```python
from build123d import *

# Parameters (mm, degrees)
BOSS_EXTRUDE1_DEPTH       = 95
SKETCH4_W                 = 5
SKETCH4_H                 = 5
BOSS_EXTRUDE4_DEPTH       = 2
FILLET1_R                 = 1.5875
F_0_80_TAPPED_HOLE1_D     = 1.19126
F_0_80_TAPPED_HOLE1_DEPTH = 4.0005
F_0_80_TAPPED_HOLE1_TIP   = 0.357890611


with BuildPart() as part:
    # Sketch1 → Boss-Extrude1 (new body)
    with BuildSketch(Plane.XY):
        Polygon((-1, 2), (-1, -2), (1, -2), (1, -0.75), (0, -0.75), (0, 0.75), (1, 0.75), (1, 2), align=None)
    extrude(amount=BOSS_EXTRUDE1_DEPTH)

    # Sketch4 → Boss-Extrude4 (add)
    with BuildSketch(Plane(origin=(1, 0, 0), x_dir=(0, 0, -1), z_dir=(1, 0, 0))):
        with Locations((-91.5, 3.25)):
            Rectangle(SKETCH4_W, SKETCH4_H)
        with Locations((-91.5, -3.25)):
            Rectangle(SKETCH4_W, SKETCH4_H)
        with Locations((-3.5, 3.25)):
            Rectangle(SKETCH4_W, SKETCH4_H)
        with Locations((-3.5, -3.25)):
            Rectangle(SKETCH4_W, SKETCH4_H)
    extrude(amount=-BOSS_EXTRUDE4_DEPTH)

    # Fillet1
    # the kernel refuses this fillet: 1.5875 mm, written as the material it adds along each edge
    with BuildSketch(Plane(origin=(1, 2, 94), x_dir=(0, 0, 1), z_dir=(-1, 0, 0))) as fillet1_piece_1:
        with BuildLine():
            CenterArc((1.5875, 1.47478812), FILLET1_R, 180, 68.279526527)
            Line((0, 1.47478812), (-0.03175, 1.47478812))
            Line((-0.03175, 1.47478812), (-0.03175, 0))
            Line((-0.03175, 0), (0, -0.03175))
            ThreePointArc((0, -0.03175), (0.5, -0.03175), (0.98825, -0.029495762))
            Line((0.98825, -0.029495762), (1, 0))
        make_face()
    extrude(amount=2)
    with BuildSketch(Plane(origin=(-1, 2, 89), x_dir=(0, 1, 0), z_dir=(1, 0, 0)), Plane(origin=(-1, 2, 6), x_dir=(0, 0, 1), z_dir=(1, 0, 0))) as fillet1_piece_2:
        with BuildLine():
            CenterArc((FILLET1_R, -FILLET1_R), FILLET1_R, 90, 90)
            Line((0, -FILLET1_R), (-FILLET1_R * 0.02, -FILLET1_R))
            Line((-FILLET1_R * 0.02, -FILLET1_R), (-FILLET1_R * 0.02, FILLET1_R * 0.02))
            Line((-FILLET1_R * 0.02, FILLET1_R * 0.02), (FILLET1_R, FILLET1_R * 0.02))
            Line((FILLET1_R, FILLET1_R * 0.02), (FILLET1_R, 0))
        make_face()
    extrude(amount=2)
    with BuildSketch(Plane(origin=(1, 2, 1), x_dir=(0, 1, 0), z_dir=(-1, 0, 0))) as fillet1_piece_3:
        with BuildLine():
            CenterArc((1.47478812, 1.5875), FILLET1_R, 201.720473473, 68.279526527)
            Line((0, 1), (-0.029495762, 0.98825))
            ThreePointArc((-0.029495762, 0.98825), (-0.03175, 0.5), (-0.03175, 0))
            Line((-0.03175, 0), (0, -0.03175))
            Line((0, -0.03175), (1.47478812, -0.03175))
            Line((1.47478812, -0.03175), (1.47478812, 0))
        make_face()
    extrude(amount=2)
    with BuildSketch(Plane(origin=(1, -2, 6), x_dir=(0, -1, 0), z_dir=(-1, 0, 0)), Plane(origin=(1, -2, 89), x_dir=(0, 0, -1), z_dir=(-1, 0, 0))) as fillet1_piece_4:
        with BuildLine():
            CenterArc((FILLET1_R, FILLET1_R), FILLET1_R, 180, 90)
            Line((0, FILLET1_R), (-FILLET1_R * 0.02, FILLET1_R))
            Line((-FILLET1_R * 0.02, FILLET1_R), (-FILLET1_R * 0.02, -FILLET1_R * 0.02))
            Line((-FILLET1_R * 0.02, -FILLET1_R * 0.02), (FILLET1_R, -FILLET1_R * 0.02))
            Line((FILLET1_R, -FILLET1_R * 0.02), (FILLET1_R, 0))
        make_face()
    extrude(amount=2)
    with BuildSketch(Plane(origin=(-1, -2, 1), x_dir=(0, 0, -1), z_dir=(1, 0, 0))) as fillet1_piece_5:
        with BuildLine():
            CenterArc((1.5875, -1.47478812), FILLET1_R, 111.720473473, 68.279526527)
            Line((0, -1.47478812), (-0.03175, -1.47478812))
            Line((-0.03175, -1.47478812), (-0.03175, 0))
            Line((-0.03175, 0), (0, 0.03175))
            ThreePointArc((0, 0.03175), (0.5, 0.03175), (0.98825, 0.029495762))
            Line((0.98825, 0.029495762), (1, 0))
        make_face()
    extrude(amount=2)
    with BuildSketch(Plane(origin=(-1, -2, 94), x_dir=(0, -1, 0), z_dir=(1, 0, 0))) as fillet1_piece_6:
        with BuildLine():
            CenterArc((1.47478812, -1.5875), FILLET1_R, 90, 68.279526527)
            Line((0, -1), (-0.029495762, -0.98825))
            ThreePointArc((-0.029495762, -0.98825), (-0.03175, -0.5), (-0.03175, 0))
            Line((-0.03175, 0), (0, 0.03175))
            Line((0, 0.03175), (1.47478812, 0.03175))
            Line((1.47478812, 0.03175), (1.47478812, 0))
        make_face()
    extrude(amount=2)

    # #0-80 Tapped Hole1
    with Locations(Plane(origin=(1, 0, 0), x_dir=(0, 0, -1), z_dir=(1, 0, 0))):
        with Locations((-91.5, 3.25), (-3.5, -3.25), (-91.5, -3.25), (-3.5, 3.25)):
            Hole(F_0_80_TAPPED_HOLE1_D / 2, depth=F_0_80_TAPPED_HOLE1_DEPTH)
            with Locations((0, 0, -(F_0_80_TAPPED_HOLE1_DEPTH + F_0_80_TAPPED_HOLE1_TIP / 2))):  # 118° drill point
                Cone(0, F_0_80_TAPPED_HOLE1_D / 2, F_0_80_TAPPED_HOLE1_TIP, mode=Mode.SUBTRACT)


solid = part.part
```
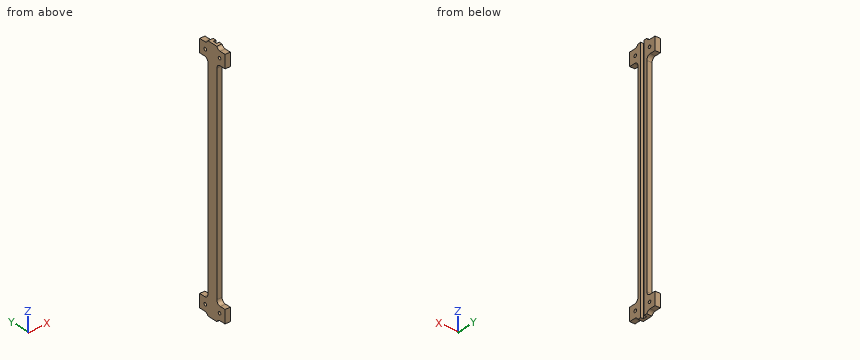
Could you check a few things on this model? Use its own coordinates, in mm. Give positions to 0.01 mm unless a question says otherwise; leave off trailing zeros. Loops run counter-clockwise (first coordinate to the right, second up) from the corner with the lowest first, then second, coordinate; pieces in that order, holes last. Notation, with made-up numbers: (10.25, 7) - (53.25, 7) arc R20 cw to (53.25, 45) - close; hole circle Ø11 at (-26.5, 28.25). An arc over 180 degrees is marked (long way). Answer in a Markdown table with one row per item. Add a question column.
Q1. Please list where these lines run through material, in increasing order: L1, parallel to Y at x = -0.45, z = 3.5; L2, parallel to Z at x = -0.45, y = 4.5; L3, parallel to Y at x = 0.4, z = 3.5. Write a range as from..to.
Q2. If we section it at A-A (x = 0.45): State how many separate pieces and enclosed holes the cut face has, plus the area to 3 significant figures.
Q3. For pin 1 (0.8 mm diameter, centred on x = 0.5, z = 56, fed in from +Y); pin 2 (1 mm diameter, centred on x = 0, y = 4.5, fed in from -Z); pin 3 (0.8 mm diameter, centred on y = 0, z = 25, fed in from +X), each with a flat end and sliding along its axis, tell me the tip position at first contact or that it passes through.
Q4. If we section it at B-B (z = 34): List the corners of the cut face in (x, y) for me.
The answers:
| question | item | result |
|---|---|---|
| 1 | L1 | y = -5.75..-3.85, -2.65..2.65, 3.85..5.75 |
| 1 | L2 | z = 1..6, 89..94 |
| 1 | L3 | y = -5.75..-3.85, -2.65..-0.75, 0.75..2.65, 3.85..5.75 |
| 2 | separate pieces | 2 |
| 2 | enclosed holes | 4 |
| 2 | area | 312 mm^2 |
| 3 | pin 1 | stops at y = 2 |
| 3 | pin 2 | stops at z = 1 |
| 3 | pin 3 | stops at x = 0 |
| 4 | outline | (-1, -2) - (1, -2) - (1, -0.75) - (0, -0.75) - (0, 0.75) - (1, 0.75) - (1, 2) - (-1, 2) - close |
